```python
from build123d import *


# Read off the part's stored shape, not the designer's step: M2.5 Machine Threads Stud1
with BuildPart() as part:
    # Sketch1 → Revolve1 (revolve)
    with BuildSketch(Plane(origin=(0, 0, 0), x_dir=(0, 0, -1), z_dir=(1, 0, 0))):
        with BuildLine():
            Line((0, 1.49), (51.9, 1.49))
            Line((51.9, 1.49), (51.9, 0))
            Line((51.9, 0), (0, 0))
            Line((0, 0), (-2.5, 0))
            ThreePointArc((-2.5, 0), (-1.767766953, 1.767766953), (0, 2.5))
            Line((0, 2.5), (0, 1.49))
        make_face()
    revolve(axis=Axis((0, 0, 65.917114172), (0, 0, -1)))

    # M2.5 Machine Threads Stud1 outline → M2.5 Machine Threads Stud1 (revolve, cut)
    with BuildSketch(Plane.XZ):
        Polygon((0.9965, -51.9), (1.49, -51.9), (1.49, -50.4), (1.25, -50.4), (1.25, -51.6465), align=None)
    revolve(axis=Axis((0, 0, 0), (0, 0, 1)), mode=Mode.SUBTRACT)


solid = part.part
```
Geometry check sheet. Reference: the model listing, model coordinates, mm. A direction names the side the tool comes from. Coordinates: 2 decimals unless noted, no trailing zeros. Order: outer loops, then holes, each group sorted by start corner. A loop starts at its lowest first (then second) coordinate and runs counter-clockwise, first axis right, second up. Notation, with made-up numbers: (-7, -23) - (20, -23) arc R29 cw to (20, 13) - close; hole circle Ø2 at (84.25, 69.5). An arc over 180 degrees is marked (long way). Answer as a JSON object with one key per item and string values. Group by question number.
Item 1: Sectioned sample at A-A, the plane y = 0. Record the cut outline in (x, z), and give its area (3 significant figures).
Item 2: Depth check by flat-ended pin: pin 1 Ø2 at (x, z) = (0, -20.5) entering from -Y; pin 2 Ø1.5 at (x, y) = (1, -2) entering from +Z. Enter the tip coordinate at first touch or a pass-through.
Item 3: Scan lines: probe 1 along Z at (x, y) = (-2.2, -0.65); probe 2 along Z at (x, y) = (0.5, -2.1); probe 3 along X at (y, z) = (1.1, -11). Record each from-to range of solid material in increasing order.
Item 4: Tool access check on faces 1 (the face through (0, 0, -51.9)), 2 (the face through (-0.27, -1.22, -51.03)). Record the directions out of +Z, -Z, +X, -X, +Y, -Y that give a thin tool (end or side, any length) a straight path to the whole face; none if there is none.
Item 5: Sectioned sample at C-C, the plane z = -3. Record the cut outline in (x, y).
Resolved:
{
 "1": {"outline": "(-2.5, 0) - (-1.49, 0) - (-1.49, -50.4) - (-1.25, -50.4) - (-1.25, -51.65) - (-1, -51.9) - (1, -51.9) - (1.25, -51.65) - (1.25, -50.4) - (1.49, -50.4) - (1.49, 0) - (2.5, 0) arc R2.5 ccw to start", "area": "164 mm^2"},
 "2": {"pin 1": "y = -1.49", "pin 2": "z = 2.01"},
 "3": {"probe 1": "0 to 0.99", "probe 2": "0 to 1.26", "probe 3": "-1.01 to 1.01"},
 "4": {"face 1": "-Z, +X, -X, +Y, -Y", "face 2": "-Z"},
 "5": {"outline": "circle Ø2.98 at (0, 0)"}
}
